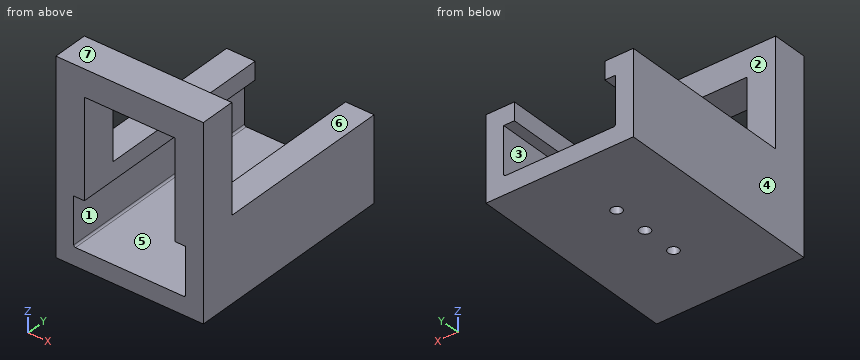
```python
from build123d import *

# Parameters (mm, degrees)
BOSS_EXTRUDE1_DEPTH = 50
BOSS_EXTRUDE2_START = 10
BOSS_EXTRUDE2_DEPTH = 10
CUT_EXTRUDE1_REACH  = 78.086
SKETCH3_R           = 1.5


with BuildPart() as part:
    # Sketch1 → Boss-Extrude1 (new body)
    with BuildSketch(Plane(origin=(0, 0, 0), x_dir=(1, 0, 0), z_dir=(0, 1, 0))):
        with BuildLine():
            Line((15.6765625, 0), (15.6765625, 12.99375))
            ThreePointArc((15.6765625, 12.99375), (15.530115891, 13.347303391), (15.1765625, 13.49375))
            Line((15.1765625, 13.49375), (-15.1765625, 13.49375))
            ThreePointArc((-15.1765625, 13.49375), (-15.530115891, 13.347303391), (-15.6765625, 12.99375))
            Line((-15.6765625, 12.99375), (-15.6765625, 0))
            Line((-15.6765625, 0), (-12.6765625, 0))
            Line((-12.6765625, 0), (-12.6765625, -5))
            Line((-12.6765625, -5), (-20.6765625, -5))
            Line((-20.6765625, -5), (-20.6765625, 0))
            Line((-20.6765625, 0), (-20.6765625, 18.49375))
            Line((-20.6765625, 18.49375), (20.6765625, 18.49375))
            Line((20.6765625, 18.49375), (20.6765625, 0))
            Line((20.6765625, 0), (20.6765625, -5))
            Line((20.6765625, -5), (12.6765625, -5))
            Line((12.6765625, -5), (12.6765625, 0))
            Line((12.6765625, 0), (15.6765625, 0))
        make_face()
    extrude(amount=BOSS_EXTRUDE1_DEPTH)

    # Sketch2 → Boss-Extrude2 (add)
    with BuildSketch(Plane.XZ.offset(BOSS_EXTRUDE2_START)):
        Polygon((-20.6765625, -18.49375), (-20.6765625, 5), (-20.6765625, 35), (20.6765625, 35), (20.6765625, 5), (20.6765625, -18.49375), align=None)
        with BuildLine():
            Line((-12.6765625, 5), (-12.6765625, 0))
            Line((-12.6765625, 0), (-15.6765625, 0))
            Line((-15.6765625, 0), (-15.6765625, -12.99375))
            ThreePointArc((-15.6765625, -12.99375), (-15.530115891, -13.347303391), (-15.1765625, -13.49375))
            Line((-15.1765625, -13.49375), (15.1765625, -13.49375))
            ThreePointArc((15.1765625, -13.49375), (15.530115891, -13.347303391), (15.6765625, -12.99375))
            Line((15.6765625, -12.99375), (15.6765625, 0))
            Line((15.6765625, 0), (12.6765625, 0))
            Line((12.6765625, 0), (12.6765625, 5))
            Line((12.6765625, 5), (12.6765625, 27.5))
            Line((12.6765625, 27.5), (-12.6765625, 27.5))
            Line((-12.6765625, 27.5), (-12.6765625, 5))
        make_face(mode=Mode.SUBTRACT)
    extrude(amount=-BOSS_EXTRUDE2_DEPTH)

    # Sketch3 → Cut-Extrude1 (cut, up to next)
    with BuildSketch(Plane(origin=(0, 0, -18.49375), x_dir=(-1, 0, 0), z_dir=(0, 0, -1)), mode=Mode.PRIVATE) as cut_extrude1_sk1:
        with Locations((0, 10)):
            Circle(SKETCH3_R)
    cut_extrude1_tool1 = extrude(cut_extrude1_sk1.sketch, amount=-CUT_EXTRUDE1_REACH, mode=Mode.PRIVATE) & part.part
    # Sketch3 → Cut-Extrude1 (cut, up to next)
    with BuildSketch(Plane(origin=(0, 0, -18.49375), x_dir=(-1, 0, 0), z_dir=(0, 0, -1)), mode=Mode.PRIVATE) as cut_extrude1_sk2:
        with Locations((0, 20)):
            Circle(SKETCH3_R)
    cut_extrude1_tool2 = extrude(cut_extrude1_sk2.sketch, amount=-CUT_EXTRUDE1_REACH, mode=Mode.PRIVATE) & part.part
    # Sketch3 → Cut-Extrude1 (cut, up to next)
    with BuildSketch(Plane(origin=(0, 0, -18.49375), x_dir=(-1, 0, 0), z_dir=(0, 0, -1)), mode=Mode.PRIVATE) as cut_extrude1_sk3:
        with Locations((0, 30)):
            Circle(SKETCH3_R)
    cut_extrude1_tool3 = extrude(cut_extrude1_sk3.sketch, amount=-CUT_EXTRUDE1_REACH, mode=Mode.PRIVATE) & part.part
    add(cut_extrude1_tool1.solids().sort_by_distance((0, 10, -18.49375))[0], mode=Mode.SUBTRACT)
    add(cut_extrude1_tool2.solids().sort_by_distance((0, 20, -18.49375))[0], mode=Mode.SUBTRACT)
    add(cut_extrude1_tool3.solids().sort_by_distance((0, 30, -18.49375))[0], mode=Mode.SUBTRACT)


solid = part.part
```
The listing builds one solid part. Answer for the finished solid, in the listing's coordinates (mm). Face numbers are marked on the shaded views. A direction names the side the tool comes from. Round coordinates to 2 decimals unless told otherwise and drop trailing zeros. Order: outer loops, then holes, each group sorted by start corner. A loop starts at its lowest first (then second) coordinate and runs counter-clockwise, first axis right, second up. Notation, with made-up numbers: (66.5, 74) -> (119.5, 74) arc R23 cw to (119.5, 108) -> close; hole circle Ø3 at (-34, 0.5). An arc over 180 degrees is marked (long way). Answer as CSV lines item,"result". Start each with the question number.
(1) The part is cut by section B-B (x = 9). Determine the outline of the cut face in (y, z), then the cut area to 3 significant figures.
(2) A tool of negligible diameter and unlimited length cuts with its end or side. For the marked faces 5, 6 and 7, from which of +Z, -Z, +X, -X, +Y, -Y can it reach the whole face along a straight path? Write none if from no direction.
(3) The part is cut by section D-D (x = 0). Determine the outline of the cut face in (y, z), then the cut area to 3 significant figures.
(4) Flat-ended cylindrical pins translate along their axes: pin 1 Ø5 at (x, y) = (0, 20) entering from +Z; pin 2 Ø2.5 at (x, y) = (18.5, 14) entering from +Z. Find the tip coordinate at first contact, or state that the pin passes through.
(5) The part is cut by section C-C (y = 20). Determine the outline of the cut face in (x, z).
(6) For a pull along X with two mould halves and no side action, classify the marked faces 1, 2, 3 and 4 as +X half, -X half, draft (parallel to the pull), parting line (faces both ways), or undercut.
(7) Find the intervals of material crossed by probe 1 along Y at (x, z) = (0, -15); probe 2 along Z at (x, y) = (15, 16); probe 3 along Z at (x, y) = (8.5, -6), in increasing order. Write a range as from..to.
(8) The part is cut by section A-A (z = -6). Determine the outline of the cut face in (x, y).
Evaluation:
1,outline,"(-10, -18.49) -> (50, -18.49) -> (50, -13.49) -> (-10, -13.49) -> close; (-10, 27.5) -> (0, 27.5) -> (0, 35) -> (-10, 35) -> close"
1,area,"375 mm²"
2,face 5,"+Y, -Y"
2,face 6,"+Z, +X, -X, +Y"
2,face 7,"+Z, +X, -X, +Y, -Y"
3,outline,"(-10, -18.49) -> (8.5, -18.49) -> (8.5, -13.49) -> (-10, -13.49) -> close; (-10, 27.5) -> (0, 27.5) -> (0, 35) -> (-10, 35) -> close; (11.5, -18.49) -> (18.5, -18.49) -> (18.5, -13.49) -> (11.5, -13.49) -> close; (21.5, -18.49) -> (28.5, -18.49) -> (28.5, -13.49) -> (21.5, -13.49) -> close; (31.5, -18.49) -> (50, -18.49) -> (50, -13.49) -> (31.5, -13.49) -> close"
3,area,"330 mm²"
4,pin 1,"z = -13.49"
4,pin 2,"z = 5"
5,outline,"(-20.68, -18.49) -> (-1.5, -18.49) -> (-1.5, -13.49) -> (-15.18, -13.49) arc R0.5 cw to (-15.68, -12.99) -> (-15.68, 0) -> (-12.68, 0) -> (-12.68, 5) -> (-20.68, 5) -> close; (1.5, -18.49) -> (20.68, -18.49) -> (20.68, 5) -> (12.68, 5) -> (12.68, 0) -> (15.68, 0) -> (15.68, -12.99) arc R0.5 cw to (15.18, -13.49) -> (1.5, -13.49) -> close"
6,face 1,"undercut"
6,face 2,"draft"
6,face 3,"undercut"
6,face 4,"-X half"
7,probe 1,"-10..8.5, 11.5..18.5, 21.5..28.5, 31.5..50"
7,probe 2,"-18.49..-13.49, 0..5"
7,probe 3,"-18.49..-13.49, 27.5..35"
8,outline,"(-20.68, -10) -> (-15.68, -10) -> (-15.68, 50) -> (-20.68, 50) -> close; (15.68, -10) -> (20.68, -10) -> (20.68, 50) -> (15.68, 50) -> close"
